```python
from build123d import *
from build123d.topology import SkipClean

# Parameters (mm, degrees)
SKETCH1_W           = 72
SKETCH1_H           = 10
BOSS_EXTRUDE1_DEPTH = 35
SKETCH2_W           = 72
SKETCH2_H           = 4
CUT_EXTRUDE1_DEPTH  = 5
SKETCH3_W           = 30
SKETCH3_H           = 8
BOSS_EXTRUDE3_DEPTH = 50
SKETCH5_R           = 15
SKETCH5_R_2         = 6
EXTRUDE_THIN1_DEPTH = 13
CUT_EXTRUDE2_START  = -13
CUT_EXTRUDE2_DEPTH  = 13
FILLET2_R           = 15
RIB12_REACH         = 88.145
SKETCH7_WALL_W      = 219.941301276
SKETCH7_WALL_H      = 10
RIB12_DRAFT_ANGLE   = 2
FILLET3_R           = 12
SKETCH9_R           = 5.1
CUT_EXTRUDE5_DEPTH  = 5


with BuildPart() as part:
    # Sketch1 → Boss-Extrude1 (new body)
    with BuildSketch(Plane.XY):
        Rectangle(SKETCH1_W, SKETCH1_H)
    extrude(amount=BOSS_EXTRUDE1_DEPTH)

    # Sketch2 → Cut-Extrude1 (cut)
    with BuildSketch(Plane.XY.offset(35)):
        with Locations((0, 3)):
            Rectangle(SKETCH2_W, SKETCH2_H)
    extrude(amount=-CUT_EXTRUDE1_DEPTH, mode=Mode.SUBTRACT)

    # Sketch3 → Boss-Extrude3 (add)
    with BuildSketch(Plane(origin=(0, 5, 0), x_dir=(1, 0, 0), z_dir=(0, 1, 0))):
        with Locations((0, -26)):
            Rectangle(SKETCH3_W, SKETCH3_H)
    extrude(amount=BOSS_EXTRUDE3_DEPTH)

    # Sketch5 → Extrude-Thin1 (add)
    with BuildSketch(Plane(origin=(0, 0, 22), x_dir=(-1, 0, 0), z_dir=(0, 0, -1))):
        with Locations((0, 55)):
            Circle(SKETCH5_R)
        with Locations((0, 55)):
            Circle(SKETCH5_R_2, mode=Mode.SUBTRACT)
    extrude(amount=-EXTRUDE_THIN1_DEPTH)

    # Sketch6 → Cut-Extrude2 (cut)
    with SkipClean():  # the faces are left unmerged after this step: merging them gives an invalid solid
        with BuildSketch(Plane.XY.offset(30).offset(CUT_EXTRUDE2_START)):
            with BuildLine():
                Line((6, 55), (-6, 55))
                ThreePointArc((-6, 55), (0, 49), (6, 55))
            make_face()
        extrude(amount=CUT_EXTRUDE2_DEPTH, mode=Mode.SUBTRACT)

    # Fillet2
    fillet2_edges = [part.edges().sort_by_distance(p)[0] for p in [
        (-15, 5, 26),
        (15, 5, 26),
    ]]
    fillet(fillet2_edges, radius=FILLET2_R)

    # Sketch7 wall → Rib12 (add, up to next)
    with BuildSketch(Plane(origin=(0, 25, 11), x_dir=(0, 0.876215908677, 0.481918749772), z_dir=(0, -0.481918749772, 0.876215908677)), mode=Mode.PRIVATE) as rib12_sk1:
        Rectangle(SKETCH7_WALL_W, SKETCH7_WALL_H)
    rib12_tool1 = extrude(rib12_sk1.sketch, amount=RIB12_REACH, mode=Mode.PRIVATE) - part.part
    add(rib12_tool1.solids().sort_by_distance((0, 25, 11))[0])

    # Rib12 draft
    rib12_draft_faces = [part.faces().sort_by_distance(p)[0] for p in [
        (-5, 24.759040625, 11.438107954),
        (5, 24.759040625, 11.438107954),
    ]]
    draft(rib12_draft_faces, Plane(origin=(0, 25, 11), x_dir=(0, 0.876215908677, 0.481918749772), z_dir=(0, 0.481918749772, -0.876215908677)), RIB12_DRAFT_ANGLE)

    # Fillet3
    fillet3_edges = [part.edges().sort_by_distance(p)[0] for p in [
        (-36, 0, 0),
        (36, 0, 0),
    ]]
    fillet(fillet3_edges, radius=FILLET3_R)

    # Sketch9 → Cut-Extrude5 (cut, symmetric)
    with SkipClean():  # the faces are left unmerged after this step: merging them gives an invalid solid
        with BuildSketch(Plane(origin=(0, 0, 0), x_dir=(1, 0, 0), z_dir=(0, 1, 0))):
            with Locations(Location((-24, -12, 0), (0, 0, 270))):
                Circle(SKETCH9_R)
            with Locations(Location((24, -12, 0), (0, 0, 270))):
                Circle(SKETCH9_R)
        extrude(amount=CUT_EXTRUDE5_DEPTH, both=True, mode=Mode.SUBTRACT)


solid = part.part
```
Geometry check sheet. Reference: the model listing, model coordinates, mm. A direction names the side the tool comes from. Give positions to 0.01 mm unless a question says otherwise; leave off trailing zeros. Loops run counter-clockwise (first coordinate to the right, second up) from the corner with the lowest first, then second, coordinate; pieces in that order, holes last. Notation, with made-up numbers: (21.5, 19.25) - (28.5, 19.25) arc R13 ccw to (28.5, 35.25) - close; hole circle Ø8 at (68, 7). An arc over 180 degrees is marked (long way). Use CSV: the item, a comma, the result in double quotes. Start each with the question number.
Q1. Release check for a two-part mould opening along Y. For faces 1 (the face through (-36, 0, 23)), 2 (the face through (-3, 18, 30)), 3 (the face through (19.51, 9.28, 25.94)) record: +Y half, -Y half, draft (parallel to the pull), parting line (faces both ways), or undercut.
Q2. Go/stop test with flat-tipped pins: pin 1 Ø2.5 at (y, z) = (29.5, 25.5) entering from +X; pin 2 Ø5 at (x, y) = (-16, 41) entering from -Z; pin 3 Ø2.5 at (y, z) = (29.5, 24.5) entering from -X; pin 4 Ø6 at (x, z) = (-24, 12) entering from +Y. Record where each tip stops, or that it passes through.
Q3. Section check D-D, the plane x = -21. Record the cut outline in (y, z), and give its area (3 significant figures).
Q4. Section check B-B, the plane z = 10. Record the cut outline in (x, y), and give its area (3 significant figures).
Q5. Section check A-A, the plane x = 0. Record the cut outline in (y, z).
Q6. Section check C-C, the plane y = 11.5. Record the cut outline in (x, z) (3 decimals), and give its area (3 significant figures).
Q7. Access from +Z, -Z, +X, -X, +Y, -Y to the whole of each face (thin tool, end or side, straight path). Record for faces 4 (the face through (-1, 1, 33)), 5 (the face through (1.953, 69.872, 29.853)), 6 (the face through (-15, 37, 26)), 7 (the face through (-17, 5, 11)).
Q8. Scan lines: probe 1 along X at (y, z) = (-1, 12); probe 2 along X at (y, z) = (55, 25); probe 3 along Y at (x, z) = (-12.5, 18.5). Record each from-to range of solid material in increasing order. Write a range as from..to.
Findings below:
1,face 1,"draft"
1,face 2,"undercut"
1,face 3,"+Y half"
2,pin 1,"stops at x = 15"
2,pin 2,"stops at z = 22"
2,pin 3,"stops at x = -15"
2,pin 4,"passes through"
3,outline,"(-5, 0) - (5, 0) - (5, 7.88) - (-5, 7.88) - close; (-5, 16.12) - (5, 16.12) - (5, 22) - (8, 22) - (8, 30) - (1, 30) - (1, 35) - (-5, 35) - close"
3,area,"272 mm^2"
4,outline,"(-35.83, -5) - (-28.69, -5) - (-28.69, 5) - (-35.83, 5) - close; (-19.31, -5) - (19.31, -5) - (19.31, 5) - (5.31, 5) - (5, 23.18) - (-5, 23.18) - (-5.31, 5) - (-19.31, 5) - close; (28.69, -5) - (35.83, -5) - (35.83, 5) - (28.69, 5) - close"
4,area,"716 mm^2"
5,outline,"(-5, 0) - (5, 0) - (45, 22) - (49, 22) - (49, 35) - (40, 35) - (40, 30) - (1, 30) - (1, 35) - (-5, 35) - close; (61, 22) - (70, 22) - (70, 35) - (61, 35) - close"
6,outline,"(-17.641, 22) - (-5.564, 22) - (-5, 3.575) - (5, 3.575) - (5.564, 22) - (17.641, 22) - (17.641, 30) - (-17.641, 30) - close"
6,area,"477 mm^2"
7,face 4,"+Z, +X, -X"
7,face 5,"+Z"
7,face 6,"+Z, -Z, -X, +Y"
7,face 7,"-Z, -X, +Y"
8,probe 1,"x = -36..-29.1, -18.9..18.9, 29.1..36"
8,probe 2,"x = -15..-6, 6..15"
8,probe 3,"y = -5..5"
